The listing builds one solid part. Answer for the finished solid, in the listing's coordinates (mm). A direction names the side the tool comes from. Round coordinates to 2 decimals unless told otherwise and drop trailing zeros. Write each loop counter-clockwise with the first axis right and the second up, starting at its lowest first coordinate (ties: lowest second). Pieces come first, ordered by that corner, then holes. Notation, with made-up numbers: M 9,68 L 23,68 A29 ccw 23,96 Z; hole C -37.75,7 d7. An arc over 180 degrees is marked long. One line per item, written item: value. Start each with the question number.
(1) Section C-C (x = 161) is taken. Determine the outline of the cut face in (y, z) (3 decimals), plus the area to 3 significant figures.
(2) Consider probe 1 along X at (y, z) = (0.5, 13.5); probe 2 along X at (y, z) = (1, 12); probe 3 along X at (y, z) = (1.5, 20). Determine where each line is inside the solid, lowest interval first.
(3) For faces 1 (the flat face through (129.37, 1.61, 2.9)), 2 (the cylindrical face through (1, 2, 48)), determine the directions among +Z, -Z, +X, -X, +Y, -Y from which every point of the face is accessible in a straight line to the end or side of a thin tool.
(4) Section B-B (y = 2.65) is taken. State how many separate pieces and enclosed holes the cut face has, plus the area to 3 significant figures.
(5) Given P1, Ø1, axis at x = 129.5, y = 1.5, coming from the +Z side; P2, Ø1, axis at y = 2, z = 15.5, coming from the -X side, each flat-ended and moving along its own axis, determine where each tip first touches the part or whether it passes through.
(6) Section A-A (x = 18) is taken. Determine the outline of the cut face in (y, z) (3 decimals).
(7) Section D-D (x = 50) is taken. Determine the outline of the cut face in (y, z) (3 decimals).
(8) For a pull along Z with two mould halves and no side action, classify faces 3 (the cylindrical face through (18, 2, 55)), 4 (the cylindrical face through (80.909, 1.61, 31.326)), 5 (the cylindrical face through (207.15, 1.61, 3.01)) as released by +Z, released by -Z, zero draft, split by the parting line, or undercut.
```python
from build123d import *

# Parameters (mm, degrees)
SKETCH1_W           = 210
SKETCH1_H           = 50
SKETCH1_R           = 1.211665018
SKETCH1_R_2         = 1.165617118
SKETCH1_R_3         = 1.5
SKETCH1_R_4         = 1.25
SKETCH1_R_5         = 1.517273905
BOSS_EXTRUDE1_DEPTH = 3.175
SKETCH2_R           = 2
CUT_EXTRUDE1_DEPTH  = 10
SKETCH3_R           = 6
SKETCH3_R_2         = 0.586995366
CUT_EXTRUDE2_DEPTH  = 57.15
CUT_EXTRUDE7_DEPTH  = 10
FILLET3_R           = 5
SKETCH11_R          = 21
SKETCH11_R_2        = 2
BOSS_EXTRUDE4_DEPTH = 3.175
SKETCH12_R          = 18.78
CUT_EXTRUDE8_DEPTH  = 10
FILLET4_R           = 10


with BuildPart() as part:
    # Sketch1 → Boss-Extrude1 (new body)
    with BuildSketch(Plane(origin=(0, 0, 0), x_dir=(1, 0, 0), z_dir=(0, 1, 0))):
        with Locations((105, -25)):
            Rectangle(SKETCH1_W, SKETCH1_H)
        with Locations(Location((3.489526233, -16.787661112, 0), (0, 0, 270))):
            Circle(SKETCH1_R, mode=Mode.SUBTRACT)
        with Locations(Location((34.37258772, -17.194005245, 0), (0, 0, 270))):
            Circle(SKETCH1_R_2, mode=Mode.SUBTRACT)
        with Locations(Location((37.520749958, -44.921198121, 0), (0, 0, 270))):
            Circle(SKETCH1_R_3, mode=Mode.SUBTRACT)
        with Locations(Location((118.879039361, -40.017685043, 0), (0, 0, 270))):
            Circle(SKETCH1_R_4, mode=Mode.SUBTRACT)
        with Locations(Location((112.302052499, -4.739260115, 0), (0, 0, 270))):
            Circle(SKETCH1_R_3, mode=Mode.SUBTRACT)
        with Locations(Location((168.975233936, -37.403209633, 0), (0, 0, 270))):
            Circle(SKETCH1_R_5, mode=Mode.SUBTRACT)
    extrude(amount=BOSS_EXTRUDE1_DEPTH)

    # Sketch2 → Cut-Extrude1 (cut)
    with BuildSketch(Plane(origin=(0, 3.175, 0), x_dir=(1, 0, 0), z_dir=(0, 1, 0))):
        with Locations(Location((10, -26, 0), (0, 0, 270))):
            Circle(SKETCH2_R)
        with Locations(Location((10, -42, 0), (0, 0, 270))):
            Circle(SKETCH2_R)
        with Locations(Location((26, -26, 0), (0, 0, 270))):
            Circle(SKETCH2_R)
        with Locations(Location((26, -42, 0), (0, 0, 270))):
            Circle(SKETCH2_R)
    extrude(amount=-CUT_EXTRUDE1_DEPTH, mode=Mode.SUBTRACT)

    # Sketch3 → Cut-Extrude2 (cut)
    with BuildSketch(Plane(origin=(0, 3.175, 0), x_dir=(1, 0, 0), z_dir=(0, 1, 0))):
        with Locations(Location((75.84991357, -28.1, 0), (0, 0, 270))):
            Circle(SKETCH3_R)
        with Locations(Location((140.771956051, -16, 0), (0, 0, 270))):
            Circle(SKETCH3_R)
        with Locations(Location((18, -34, 0), (0, 0, 270))):
            Circle(SKETCH3_R_2)
        with Locations(Location((197.921956051, -16, 0), (0, 0, 270))):
            Circle(SKETCH3_R)
    extrude(amount=-CUT_EXTRUDE2_DEPTH, mode=Mode.SUBTRACT)

    # Sketch10 → Cut-Extrude7 (cut)
    with BuildSketch(Plane(origin=(0, 3.175, 0), x_dir=(1, 0, 0), z_dir=(0, 1, 0))):
        Polygon((210, -27.859435908), (165.502877994, -50), (210, -50), align=None)
        Polygon((92.532613397, 0), (77.65477062, -7.402812063), (0, -7.402812063), (0, 0), align=None)
        Polygon((124.109963401, 0), (134.770313295, -5.880313872), (187.967697751, -5.880313872), (198.343585303, 0), align=None)
    extrude(amount=-CUT_EXTRUDE7_DEPTH, mode=Mode.SUBTRACT)

    # Fillet3
    fillet3_edges = [part.edges().sort_by_distance(p)[0] for p in [
        (0, 1.5875, 7.402812063),
        (0, 1.5875, 50),
        (92.532613397, 1.5875, 0),
        (210, 1.5875, 27.859435908),
        (165.502877994, 1.5875, 50),
        (77.65477062, 1.5875, 7.402812063),
    ]]
    fillet(fillet3_edges, radius=FILLET3_R)

    # Sketch11 → Boss-Extrude4 (add)
    with BuildSketch(Plane(origin=(0, 3.175, 0), x_dir=(1, 0, 0), z_dir=(0, 1, 0))):
        with Locations((18, -34)):
            Circle(SKETCH11_R)
        with Locations(Location((10, -26, 0), (0, 0, 270))):
            Circle(SKETCH11_R_2, mode=Mode.SUBTRACT)
        with Locations(Location((10, -42, 0), (0, 0, 270))):
            Circle(SKETCH11_R_2, mode=Mode.SUBTRACT)
        with Locations(Location((26, -26, 0), (0, 0, 270))):
            Circle(SKETCH11_R_2, mode=Mode.SUBTRACT)
        with Locations(Location((26, -42, 0), (0, 0, 270))):
            Circle(SKETCH11_R_2, mode=Mode.SUBTRACT)
    extrude(amount=-BOSS_EXTRUDE4_DEPTH)

    # Sketch12 → Cut-Extrude8 (cut)
    with BuildSketch(Plane(origin=(0, 3.175, 0), x_dir=(1, 0, 0), z_dir=(0, 1, 0))):
        with Locations(Location((18, -34, 0), (0, 0, 270))):
            Circle(SKETCH12_R)
    extrude(amount=-CUT_EXTRUDE8_DEPTH, mode=Mode.SUBTRACT)

    # Fillet4
    fillet4_edges = [part.edges().sort_by_distance(p)[0] for p in [
        (210, 1.5875, 0),
    ]]
    fillet(fillet4_edges, radius=FILLET4_R)


solid = part.part
```
Recorded:
1. outline: M 0,5.88 L 3.175,5.88 L 3.175,50 L 0,50 Z
1. area: 140 mm2
2. probe 1: x = 0 to 135.32, 146.23 to 192.47, 203.38 to 210
2. probe 2: x = 0.02 to 136.3, 145.24 to 193.45, 202.39 to 210
2. probe 3: x = 0 to 5.48, 30.52 to 136.3, 145.24 to 193.45, 202.39 to 210
3. face 1: -Z, +Y, -Y
3. face 2: +Z, -X, +Y, -Y
4. separate pieces: 1
4. enclosed holes: 10
4. area: 7,620 mm2
5. P1: stops at z = 50
5. P2: stops at x = 0
6. outline: M 0,7.403 L 3.175,7.403 L 3.175,15.22 L 0,15.22 Z; M 0,52.78 L 3.175,52.78 L 3.175,55 L 0,55 Z
7. outline: M 0,7.403 L 3.175,7.403 L 3.175,50 L 0,50 Z
8. face 3: released by +Z
8. face 4: undercut
8. face 5: released by -Z
